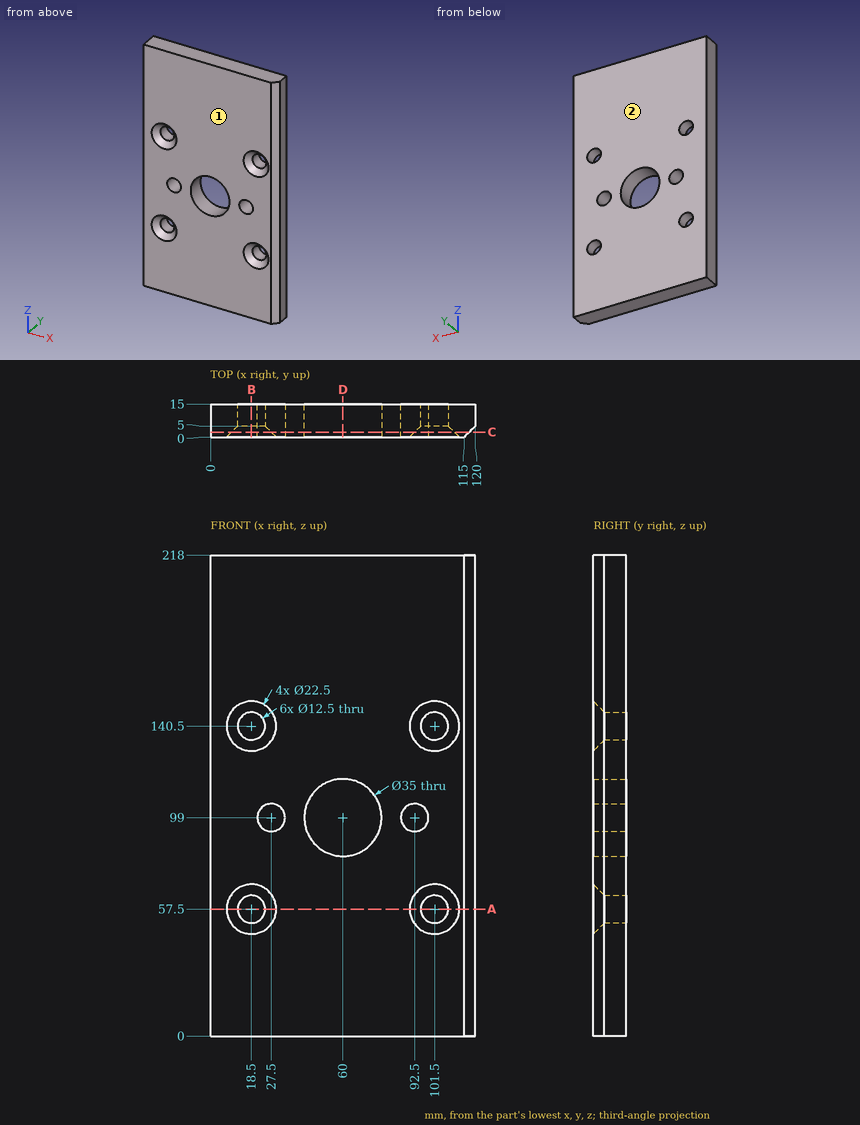
Verification items for this drawing (mm, ordinates from the low corner). Give positions to 0.01 mm unless a question says otherwise; leave off trailing zeros. Write each loop counter-clockwise with the first axis right and the second up, starting at its lowest first coordinate (ties: lowest second). Pieces come first, ordered by that corner, then holes. Notation, with made-up numbers: (45.25, 27) -> (55.25, 27) arc R30 ccw to (55.25, 54) -> close; hole circle Ø11 at (61, -37.5). An arc over 180 degrees is marked (long way). Use one line per item in the form item = value.
Item 1: Sectioned sample at C-C on y = 2.25. Enter the section's corners in (x, z).
Results list:
outline = (0, 0) -> (117.25, 0) -> (117.25, 218) -> (0, 218) -> close; hole circle Ø18 at (18.5, 57.5); hole circle Ø18 at (18.5, 140.5); hole circle Ø12.5 at (27.5, 99); hole circle Ø35 at (60, 99); hole circle Ø12.5 at (92.5, 99); hole circle Ø18 at (101.5, 57.5); hole circle Ø18 at (101.5, 140.5)
Item 2: Depth check by flat-ended pin: pin 1 Ø12 at (x, z) = (70, 135.5) entering from -Y; pin 2 Ø7.5 at (x, z) = (92.5, 99) entering from -Y; pin 3 Ø1.5 at (y, z) = (3, 111) entering from +X. Enter the tip coordinate at first touch or a pass-through.
Results list:
pin_1 = 0
pin_2 = through
pin_3 = 118.75
Item 3: Sectioned sample at A-A on z = 57.5. Enter the section's corners in (x, y), plus the area to 3 significant figures.
Results list:
outline = (0, 0) -> (7.25, 0) -> (12.25, 5) -> (12.25, 15) -> (0, 15) -> close; (24.75, 5) -> (29.75, 0) -> (90.25, 0) -> (95.25, 5) -> (95.25, 15) -> (24.75, 15) -> close; (107.75, 5) -> (112.75, 0) -> (115, 0) -> (120, 5) -> (120, 15) -> (107.75, 15) -> close
area = 1,360 mm2
Item 4: Sectioned sample at D-D on x = 60. Enter the section's corners in (y, z), plus the area to 4 significant figures.
Results list:
outline = (0, 0) -> (15, 0) -> (15, 81.5) -> (0, 81.5) -> close; (0, 116.5) -> (15, 116.5) -> (15, 218) -> (0, 218) -> close
area = 2,745 mm2
Item 5: Sectioned sample at B-B on x = 18.5. Enter the section's corners in (y, z), plus the area to 4 significant figures.
Results list:
outline = (0, 0) -> (15, 0) -> (15, 51.25) -> (5, 51.25) -> (0, 46.25) -> close; (0, 68.75) -> (5, 63.75) -> (15, 63.75) -> (15, 134.25) -> (5, 134.25) -> (0, 129.25) -> close; (0, 151.75) -> (5, 146.75) -> (15, 146.75) -> (15, 218) -> (0, 218) -> close
area = 2,845 mm2
Item 6: Scan lines: line 1 (Z direction, x = 101.5, y = 8.75); line 2 (Z direction, x = 60, y = 3.75); line 3 (X direction, y = 3, z = 98.5). Record each from-to range of solid material in increasing order.
Results list:
line_1 = 0 to 51.25, 63.75 to 134.25, 146.75 to 218
line_2 = 0 to 81.5, 116.5 to 218
line_3 = 0 to 21.27, 33.73 to 42.51, 77.49 to 86.27, 98.73 to 118
Item 7: Mould release check, pull along Y, two halves, no side actions. Record for the marked faces 1 and 2: released by +Y, released by -Y, zero draft, split by the parting line, or undercut.
Results list:
face_1 = released by -Y
face_2 = released by +Y
